Geometry: final body of the model. Coordinates: model frame, mm. A direction names the side the tool comes from. Give positions to 0.01 mm unless a question says otherwise; leave off trailing zeros. Order: outer loops, then holes, each group sorted by start corner. A loop starts at its lowest first (then second) coordinate and runs counter-clockwise, first axis right, second up. Notation, with made-up numbers: (22.5, 74.25) - (43.5, 74.25) arc R20 ccw to (43.5, 98.25) - close; hole circle Ø11 at (50, 16). An arc over 180 degrees is marked (long way). Write item = value, one per line. Start each with the question number.
from build123d import *

# Parameters (mm, degrees)
SKETCH1_W           = 45
SKETCH1_H           = 250
BOSS_EXTRUDE1_DEPTH = 12
SKETCH2_W           = 5
SKETCH2_H           = 105
CUT_EXTRUDE1_DEPTH  = 12
SKETCH3_R           = 1.75
CUT_EXTRUDE2_DEPTH  = 35
SKETCH5_W           = 5
SKETCH5_H           = 35
BOSS_EXTRUDE2_DEPTH = 12
SKETCH7_R           = 12
SKETCH7_R_2         = 1.25
CUT_EXTRUDE3_DEPTH  = 35


with BuildPart() as part:
    # Sketch1 → Boss-Extrude1 (new body)
    with BuildSketch(Plane(origin=(0, 0, 0), x_dir=(1, 0, 0), z_dir=(0, 1, 0))):
        Rectangle(SKETCH1_W, SKETCH1_H)
    extrude(amount=BOSS_EXTRUDE1_DEPTH)

    # Sketch2 → Cut-Extrude1 (cut)
    with BuildSketch(Plane(origin=(0, 12, 0), x_dir=(1, 0, 0), z_dir=(0, 1, 0))):
        with Locations((20, 37.5)):
            Rectangle(SKETCH2_W, SKETCH2_H)
        with Locations((-20, 37.5)):
            Rectangle(SKETCH2_W, SKETCH2_H)
    extrude(amount=-CUT_EXTRUDE1_DEPTH, mode=Mode.SUBTRACT)

    # Sketch3 → Cut-Extrude2 (cut)
    with BuildSketch(Plane(origin=(17.5, 0, 0), x_dir=(0, 0, -1), z_dir=(1, 0, 0))):
        with Locations((10, 6)):
            Circle(SKETCH3_R)
        with Locations((70, 6)):
            Circle(SKETCH3_R)
    extrude(amount=-CUT_EXTRUDE2_DEPTH, mode=Mode.SUBTRACT)

    # Sketch5 → Boss-Extrude2 (add)
    with BuildSketch(Plane(origin=(0, 12, 0), x_dir=(1, 0, 0), z_dir=(0, 1, 0))):
        with Locations((25, 107.5)):
            Rectangle(SKETCH5_W, SKETCH5_H)
        with Locations((-25, 107.5)):
            Rectangle(SKETCH5_W, SKETCH5_H)
    extrude(amount=-BOSS_EXTRUDE2_DEPTH)

    # Sketch7 → Cut-Extrude3 (cut)
    with BuildSketch(Plane(origin=(0, 12, 0), x_dir=(1, 0, 0), z_dir=(0, 1, 0))):
        with Locations(Location((0, 105, 0), (0, 0, 270))):
            Circle(SKETCH7_R)
        with Locations(Location((21.920310217, 105, 0), (0, 0, 270))):
            Circle(SKETCH7_R_2)
        with Locations(Location((-21.920310217, 105, 0), (0, 0, 270))):
            Circle(SKETCH7_R_2)
        with Locations(Location((0, 83.079689783, 0), (0, 0, 270))):
            Circle(SKETCH7_R_2)
    extrude(amount=-CUT_EXTRUDE3_DEPTH, mode=Mode.SUBTRACT)


solid = part.part
Q1. Set-up query: faces 5 (the flat face through (27.5, 6, -107)), 6 (the flat face through (-22.5, 6, 71)), 7 (the flat face through (22.5, 6, 71)), 8 (the flat face through (-20, 6, 15)), 9 (the flat face through (22, 6, -90)). Return all of +Z, -Z, +X, -X, +Y, -Y with unobstructed straight access to the full face (end or side cutting, diameter ignored); none if empty.
Q2. Contact query for flat-ended pins moving along their axis: pin 1 (3.5 mm diameter, centred on y = 6, z = -42, fed in from -X); pin 2 (6 mm diameter, centred on y = 2.5, z = 54, fed in from +X); pin 3 (3 mm diameter, centred on y = 10, z = -25, fed in from +X). Output: stop coordinate, or through.
Q3. Section D-D, the plane z = 74. Return the cut outline in (x, y), then the cut area to 3 significant figures.
Q4. Section A-A, the plane x = -8.5. Return the cut outline in (y, z).
Q5. Material intervals for line 1 along X through (y, z) = (6.75, -105); line 2 along Y through (x, z) = (0, -70); line 3 along X through (y, z) = (1, 63), sorted ascending. Write a range as from..to.
Q6. Section C-C, the plane z = -50.5. Return the cut outline in (x, y).
Q7. Pull-direction query (Z, two-part tool) for faces 1 (the flat face through (0, 6, 125)), 2 (the flat face through (20, 6, 15)), 3 (the flat face through (17.5, 6, -37)), 4 (the flat face through (0, 12, -2)); classes: +Z half, -Z half, draft (parallel to the pull), parting line (faces both ways), or undercut.
Q8. Section B-B, the plane y = 10. Return the cut outline in (x, z).
The answers:
q1.face_5 = +Z, -Z, +X, +Y, -Y
q1.face_6 = +Z, -X, +Y, -Y
q1.face_7 = +Z, +X, +Y, -Y
q1.face_8 = -X, +Y, -Y
q1.face_9 = +X, +Y, -Y
q2.pin_1 = -17.5
q2.pin_2 = 22.5
q2.pin_3 = 17.5
q3.outline = (-22.5, 0) - (22.5, 0) - (22.5, 12) - (-22.5, 12) - close
q3.area = 540 mm²
q4.outline = (0, -125) - (12, -125) - (12, -113.47) - (0, -113.47) - close; (0, -96.53) - (12, -96.53) - (12, 125) - (0, 125) - close; hole circle Ø3.5 at (6, -70); hole circle Ø3.5 at (6, -10)
q5.line_1 = -27.5..-23.17, -20.67..-12, 12..20.67, 23.17..27.5
q5.line_2 = 0..4.25, 7.75..12
q5.line_3 = -22.5..22.5
q6.outline = (-17.5, 0) - (17.5, 0) - (17.5, 12) - (-17.5, 12) - close
q7.face_1 = +Z half
q7.face_2 = undercut
q7.face_3 = undercut
q7.face_4 = draft
q8.outline = (-27.5, -125) - (27.5, -125) - (27.5, -90) - (17.5, -90) - (17.5, 15) - (22.5, 15) - (22.5, 125) - (-22.5, 125) - (-22.5, 15) - (-17.5, 15) - (-17.5, -90) - (-27.5, -90) - close; hole circle Ø2.5 at (-21.92, -105); hole circle Ø24 at (0, -105); hole circle Ø2.5 at (0, -83.08); hole circle Ø2.5 at (21.92, -105)
